Study the drawing (mm; zero at the part's minimum x, y, z) and answer. Give positions to 0.01 mm unless a question says otherwise; leave off trailing zeros. Write each loop counter-clockwise with the first axis right and the second up, starting at its lowest first coordinate (ties: lowest second). Pieces come first, ordered by that corner, then holes. Notation, with made-up numbers: (-39.75, 47.5) - (-35.75, 47.5) arc R22 cw to (-35.75, 83.5) - close; hole circle Ø11 at (35.5, 63.25). An arc over 180 degrees is marked (long way). Answer as CSV lines item,"result".
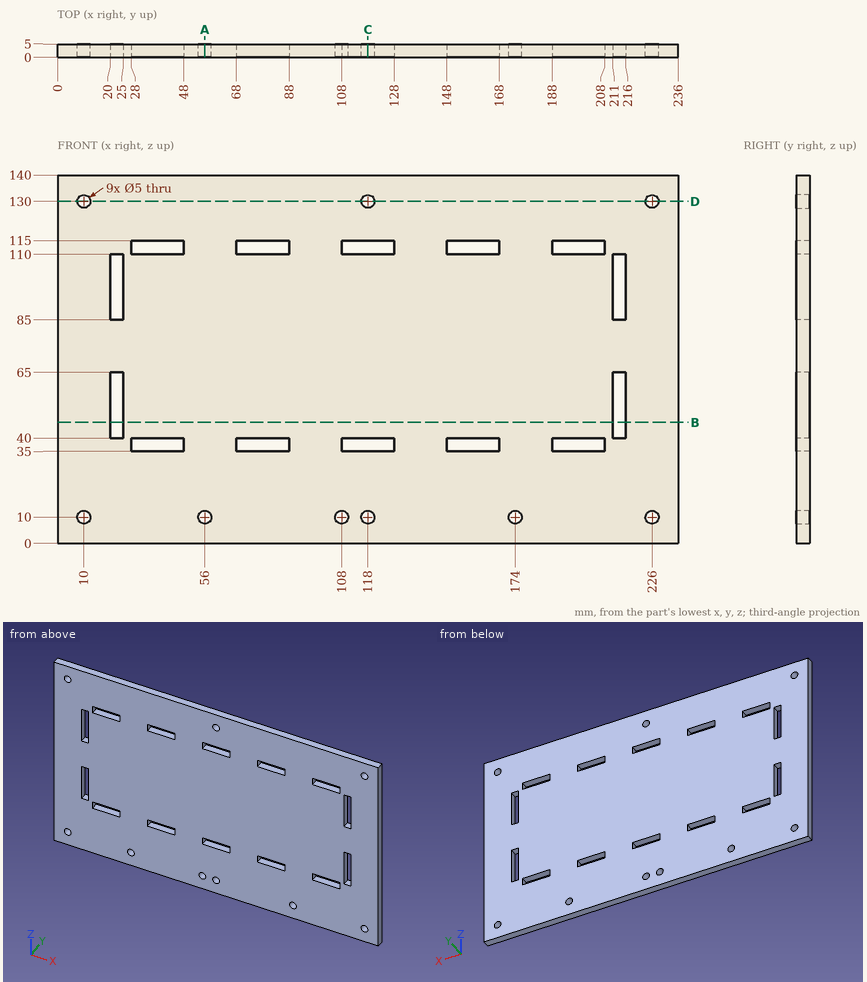
(1) Find the intervals of material crossed by L1, parallel to X at y = 2.55, z = 51.5; L2, parallel to X at y = 1.75, z = 37; L3, parallel to X at y = 1.7, z = 130, in increasing order.
Worked out:
L1,"x = 0 to 20, 25 to 211, 216 to 236"
L2,"x = 0 to 28, 48 to 68, 88 to 108, 128 to 148, 168 to 188, 208 to 236"
L3,"x = 0 to 7.5, 12.5 to 115.5, 120.5 to 223.5, 228.5 to 236"
(2) A cutting plane is placed at B-B (z = 46). Write down the section's boundary in (x, y), and give its area (3 significant figures).
Worked out:
outline,"(0, 0) - (20, 0) - (20, 5) - (0, 5) - close; (25, 0) - (211, 0) - (211, 5) - (25, 5) - close; (216, 0) - (236, 0) - (236, 5) - (216, 5) - close"
area,"1,130 mm^2"
(3) A cutting plane is placed at C-C (x = 118). Write down the section's boundary in (y, z), and give its area (3 significant figures).
Worked out:
outline,"(0, 0) - (5, 0) - (5, 7.5) - (0, 7.5) - close; (0, 12.5) - (5, 12.5) - (5, 35) - (0, 35) - close; (0, 40) - (5, 40) - (5, 110) - (0, 110) - close; (0, 115) - (5, 115) - (5, 127.5) - (0, 127.5) - close; (0, 132.5) - (5, 132.5) - (5, 140) - (0, 140) - close"
area,"600 mm^2"
(4) A cutting plane is placed at D-D (z = 130). Write down the section's boundary in (x, y).
Worked out:
outline,"(0, 0) - (7.5, 0) - (7.5, 5) - (0, 5) - close; (12.5, 0) - (115.5, 0) - (115.5, 5) - (12.5, 5) - close; (120.5, 0) - (223.5, 0) - (223.5, 5) - (120.5, 5) - close; (228.5, 0) - (236, 0) - (236, 5) - (228.5, 5) - close"
(5) A cutting plane is placed at A-A (x = 56). Write down the section's boundary in (y, z), and give its area (3 significant figures).
Worked out:
outline,"(0, 0) - (5, 0) - (5, 7.5) - (0, 7.5) - close; (0, 12.5) - (5, 12.5) - (5, 140) - (0, 140) - close"
area,"675 mm^2"
